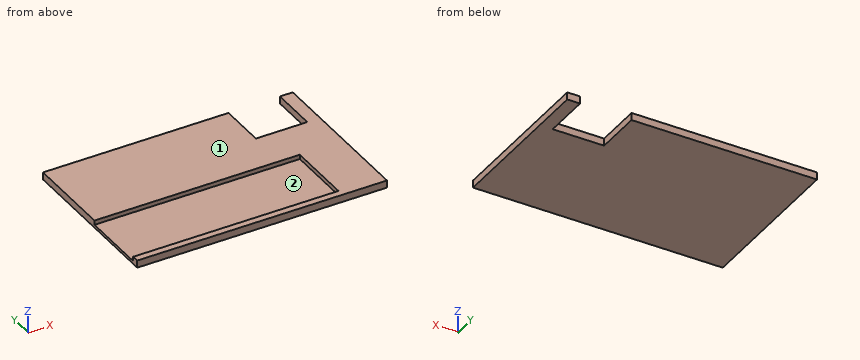
from build123d import *

# Parameters (mm, degrees)
BOSS_EXTRUDE1_DEPTH = 5
SKETCH2_W           = 140
SKETCH2_H           = 45
CUT_EXTRUDE1_DEPTH  = 3
SKETCH3_W           = 35
SKETCH3_H           = 32
CUT_EXTRUDE3_DEPTH  = 148.286881187


with BuildPart() as part:
    # Sketch1 → Boss-Extrude1 (new body)
    with BuildSketch(Plane.XY):
        Polygon((0, -2.718152765), (-101.259492884, -2.718152765), (-101.259492884, 106.840724775), (68.740507116, 106.840724775), (68.740507116, -2.718152765), align=None)
    extrude(amount=BOSS_EXTRUDE1_DEPTH)

    # Sketch2 → Cut-Extrude1 (cut)
    with BuildSketch(Plane.XY.offset(5)):
        with Locations((-31.52, 24.5)):
            Rectangle(SKETCH2_W, SKETCH2_H)
    extrude(amount=-CUT_EXTRUDE1_DEPTH, mode=Mode.SUBTRACT)

    # Sketch3 → Cut-Extrude3 (cut, through all)
    with BuildSketch(Plane.XY):
        with Locations((42.5, 91)):
            Rectangle(SKETCH3_W, SKETCH3_H)
    extrude(amount=CUT_EXTRUDE3_DEPTH, mode=Mode.SUBTRACT)


solid = part.part
Input: part model. Units: mm. Frame: model coordinates. Face numbers are marked on the shaded views. Coordinates: 2 decimals unless noted, no trailing zeros. Loops run counter-clockwise (first coordinate to the right, second up) from the corner with the lowest first, then second, coordinate; pieces in that order, holes last. Notation, with made-up numbers: (78, -9) -> (96, -9) arc R11 ccw to (96, 10) -> close; hole circle Ø1 at (-26.5, -24). An arc over 180 degrees is marked (long way). Write item = value, one per line. Start each with the question number.
Item 1: Cut plane B-B, the plane z = 1.1. Return loops of the section in (x, y).
Item 2: Cut plane C-C, the plane y = 15. Return loops of the section in (x, z), plus the area to 3 significant figures.
Item 3: Material intervals for line 1 (Y direction, x = 12, z = 4.3); line 2 (Z direction, x = -87, y = 39.5); line 3 (X direction, y = 95, z = 3.45), sorted ascending.
Item 4: Mould query, pull axis Y, two halves, no side actions, for the marked faces 1 and 2. Classes: pulls with the +Y half, pulls with the -Y half, needs draft (parallel to the pull), parting line crosses it, or undercut.
Item 5: First-contact query: P1, Ø1.5, axis at y = 28, z = 3.5, coming from the -X side; P2, Ø13.5, axis at x = -25, y = 32.5, coming from the +Z side. Flat tips, straight axial feed; report the tip coordinate or a pass-through.
Item 6: Cut plane A-A, the plane x = -49.5. Return loops of the section in (y, z).
Ans:
q1.outline = (-101.26, -2.72) -> (68.74, -2.72) -> (68.74, 106.84) -> (60, 106.84) -> (60, 75) -> (25, 75) -> (25, 106.84) -> (-101.26, 106.84) -> close
q2.outline = (-101.26, 0) -> (68.74, 0) -> (68.74, 5) -> (38.48, 5) -> (38.48, 2) -> (-101.26, 2) -> close
q2.area = 431 mm²
q3.line_1 = -2.72 to 2, 47 to 106.84
q3.line_2 = 0 to 2
q3.line_3 = -101.26 to 25, 60 to 68.74
q4.face_1 = needs draft
q4.face_2 = undercut
q5.P1 = 38.48
q5.P2 = 2
q6.outline = (-2.72, 0) -> (106.84, 0) -> (106.84, 5) -> (47, 5) -> (47, 2) -> (2, 2) -> (2, 5) -> (-2.72, 5) -> close
